from build123d import *

# Parameters (mm, degrees)
F0_R     = 54.61
F0_R_2   = 14.224
F1_DEPTH = 60.96
F2_R     = 10.16
F3_R     = 5.08
F0_R_3   = 4.7625
F4_DEPTH = 50.8


with BuildPart() as f1:
    # F0 (on Top) → F1 (new body)
    with BuildSketch(Plane.XY):
        Circle(F0_R)
        Circle(F0_R_2, mode=Mode.SUBTRACT)
    extrude(amount=F1_DEPTH)

    # F2
    f2_edges = [f1.edges().sort_by_distance(p)[0] for p in [
        (-54.61, 0, 0),
        (-54.61, 0, 60.96),
    ]]
    fillet(f2_edges, radius=F2_R)

    # F3
    f3_edges = [f1.edges().sort_by_distance(p)[0] for p in [
        (-14.224, 0, 60.96),
        (-14.224, 0, 0),
    ]]
    fillet(f3_edges, radius=F3_R)

    # F0 (on Top) → F4 (join)
    with BuildSketch(Plane.XY):
        Circle(F0_R_2)
        Circle(F0_R_3, mode=Mode.SUBTRACT)
    extrude(amount=F4_DEPTH)


solid = f1.part
Design review of the part built by this model. Coordinates are the model's own, in mm. A direction names the side the tool comes from. Give positions to 0.01 mm unless a question says otherwise; leave off trailing zeros. Loops run counter-clockwise (first coordinate to the right, second up) from the corner with the lowest first, then second, coordinate; pieces in that order, holes last. Notation, with made-up numbers: (12, 75) - (59, 75) arc R32 cw to (59, 101) - close; hole circle Ø4 at (-3, 67.25). An arc over 180 degrees is marked (long way). Write item = value, one per line.
1) To check wall thickness, follow line 1 (Y direction, x = 0, z = 37.5); line 2 (Y direction, x = 0, z = 54); line 3 (Z direction, x = 12, y = -4.5). State the ranges of each line that lie inside material, in increasing order.
Result sheet:
line_1 = -54.61 to -4.76, 4.76 to 54.61
line_2 = -54.09 to -14.22, 14.22 to 54.09
line_3 = 0 to 50.8
2) Take a section at A-A on x = 0. State the section outline as (y, z) points, and give its area (3 significant figures).
Result sheet:
outline = (-54.61, 10.16) arc R10.16 ccw to (-44.45, 0) - (-19.3, 0) arc R5.08 ccw to (-14.22, 5.08) - (-14.22, 0) - (-4.76, 0) - (-4.76, 50.8) - (-14.22, 50.8) - (-14.22, 55.88) arc R5.08 ccw to (-19.3, 60.96) - (-44.45, 60.96) arc R10.16 ccw to (-54.61, 50.8) - close; (4.76, 0) - (14.22, 0) - (14.22, 5.08) arc R5.08 ccw to (19.3, 0) - (44.45, 0) arc R10.16 ccw to (54.61, 10.16) - (54.61, 50.8) arc R10.16 ccw to (44.45, 60.96) - (19.3, 60.96) arc R5.08 ccw to (14.22, 55.88) - (14.22, 50.8) - (4.76, 50.8) - close
area = 5,770 mm2
3) Take a section at D-D on z = 52.5. State the section outline as (x, y) points.
Result sheet:
outline = circle Ø108.93 at (0, 0); hole circle Ø28.45 at (0, 0)
4) Tool access review of faces 4 (the face through (6, 0, 50.8)), 5 (the face through (19, -9, 60.96)): name each direction out of +Z, -Z, +X, -X, +Y, -Y from which nothing blocks a thin tool from reaching the whole face with its end or side.
Result sheet:
face_4 = +Z
face_5 = +Z, +X, -X, +Y, -Y
5) Clearance check with flat-ended pins moving along their axes: pin 1 Ø3 at (y, z) = (41.5, 52) entering from -X; pin 2 Ø1 at (x, z) = (-42.5, 9.5) entering from +Y; pin 3 Ø5 at (x, z) = (14.5, 11) entering from +Y; pin 4 Ø7.5 at (x, y) = (0, 0) entering from -Z. State where each tip first meets the part, or that it passes through.
Result sheet:
pin_1 = -37.09
pin_2 = 34.87
pin_3 = 53.28
pin_4 = through
6) Take a section at C-C on z = 34.5. State the section outline as (x, y) points (1 decimal), and give its area (3 significant figures).
Result sheet:
outline = circle Ø109.2 at (0, 0); hole circle Ø9.5 at (0, 0)
area = 9,300 mm2
7) Draft analysis for pull direction Y (two halves, no side actions). For faces 1 (the face through (-3.083, -13.886, 53.304)), 2 (the face through (19, -9, 0)), 3 (the face through (-7.109, 54.145, 30.196)), state which applies: +Y half, -Y half, draft (parallel to the pull), parting line (faces both ways), or undercut.
Result sheet:
face_1 = undercut
face_2 = draft
face_3 = parting line
